Read the model definition and answer for the solid it produces. Units are mm, in the model's axes. Face numbers are marked on the shaded views. A direction names the side the tool comes from. Coordinates: 2 decimals unless noted, no trailing zeros. Write each loop counter-clockwise with the first axis right and the second up, starting at its lowest first coordinate (ties: lowest second). Pieces come first, ordered by that corner, then holes. Notation, with made-up numbers: M 64,13.5 L 100,13.5 A21 ccw 100,30.5 Z; hole C -32.75,51.25 d4. An arc over 180 degrees is marked long. Use a Markdown table: item, result. Add a question column.
from build123d import *

# Parameters (mm, degrees)
SKETCH4_R                               = 5
CUT_EXTRUDE1_DEPTH                      = 106.234262481
CBORE_FOR_M8_HEX_HEAD_BOLT1_D           = 8.4
CBORE_FOR_M8_HEX_HEAD_BOLT1_DEPTH       = 28.41
CBORE_FOR_M8_HEX_HEAD_BOLT1_CBORE_D     = 18.01
CBORE_FOR_M8_HEX_HEAD_BOLT1_CBORE_DEPTH = 5.68
CBORE_FOR_M8_HEX_HEAD_BOLT1_TIP         = 2.5236146
CHAMFER1_SIZE                           = 5
SKETCH8_R                               = 10
CUT_EXTRUDE2_DEPTH                      = 15
CIRPATTERN1_COUNT                       = 9


with BuildPart() as part:
    # Sketch2 → Revolve1 (revolve)
    with BuildSketch(Plane(origin=(0, 0, 0), x_dir=(1, 0, 0), z_dir=(0, 1, 0))):
        Polygon((49, 0), (71, 0), (71, 12), (51, 12), (51, 27), (31, 27), (31, 25), (31, 9), (28, 9), (25, -13.5), (27.5, -13.5), (27.5, -26.5), (27.5, -31.5), (47, -31.5), (47, -9.5), (47, -2), (47, 0), align=None)
    revolve(axis=Axis((0, 0, 21.110532956), (0, 0, -1)))

    # Sketch4 → Cut-Extrude1 (cut, through all)
    with BuildSketch(Plane.XY):
        with Locations((29, -50.229473419)):
            Circle(SKETCH4_R)
        with Locations((29, 50.22947342)):
            Circle(SKETCH4_R)
        with Locations((-58, 0)):
            Circle(SKETCH4_R)
    extrude(amount=-CUT_EXTRUDE1_DEPTH, mode=Mode.SUBTRACT)

    # CBORE for M8 Hex Head Bolt1
    with Locations(Plane.XY):
        with Locations((-10.071594305, 57.118849675), (-44.430577701, 37.281681362), (-44.430577701, -37.281681362), (-10.071594305, -57.118849675), (54.502172006, -19.837168313), (54.502172006, 19.837168313)):
            CounterBoreHole(CBORE_FOR_M8_HEX_HEAD_BOLT1_D / 2, CBORE_FOR_M8_HEX_HEAD_BOLT1_CBORE_D / 2, CBORE_FOR_M8_HEX_HEAD_BOLT1_CBORE_DEPTH, depth=CBORE_FOR_M8_HEX_HEAD_BOLT1_DEPTH)
            with Locations((0, 0, -(CBORE_FOR_M8_HEX_HEAD_BOLT1_DEPTH + CBORE_FOR_M8_HEX_HEAD_BOLT1_TIP / 2))):  # 118° drill point
                Cone(0, CBORE_FOR_M8_HEX_HEAD_BOLT1_D / 2, CBORE_FOR_M8_HEX_HEAD_BOLT1_TIP, mode=Mode.SUBTRACT)

    # Sketch7 → Cut-Revolve1 (revolve, cut)
    with BuildSketch(Plane(origin=(0, 0, 0), x_dir=(1, 0, 0), z_dir=(0, 1, 0)), mode=Mode.PRIVATE) as cut_revolve1_sk:
        Polygon((47, -9.5), (47, -7.5), (35, -7.5), (35, -8.5), (36, -8.5), (36, -31.5), (67.825, -31.5), (67.825, -9.5), align=None)
    revolve(cut_revolve1_sk.sketch.rotate(Axis((0, 0, 7.5), (0, 0, 1)), 180), axis=Axis((0, 0, 7.5), (0, 0, 1)), mode=Mode.SUBTRACT)

    # Chamfer1
    chamfer1_edges = [part.edges().sort_by_distance(p)[0] for p in [
        (36, 0, 31.5),
    ]]
    chamfer(chamfer1_edges, length=CHAMFER1_SIZE)

    # Sketch8 → Cut-Extrude2 (cut)
    with BuildSketch(Plane(origin=(0, 0, -27), x_dir=(-1, 0, 0), z_dir=(0, 0, -1))):
        with Locations((44.430577701, 37.281681362)):
            Circle(SKETCH8_R)
    cut_extrude2 = extrude(amount=-CUT_EXTRUDE2_DEPTH, mode=Mode.SUBTRACT)

    # CirPattern1: Cut-Extrude2 ×9 about axis, 3 skipped
    cirpattern1_axis = Axis((0, 0, -12), (0, 0, 1))
    add([cut_extrude2.rotate(cirpattern1_axis, i * 360 / CIRPATTERN1_COUNT) for i in range(1, CIRPATTERN1_COUNT) if i not in (1, 4, 7)], mode=Mode.SUBTRACT)


solid = part.part
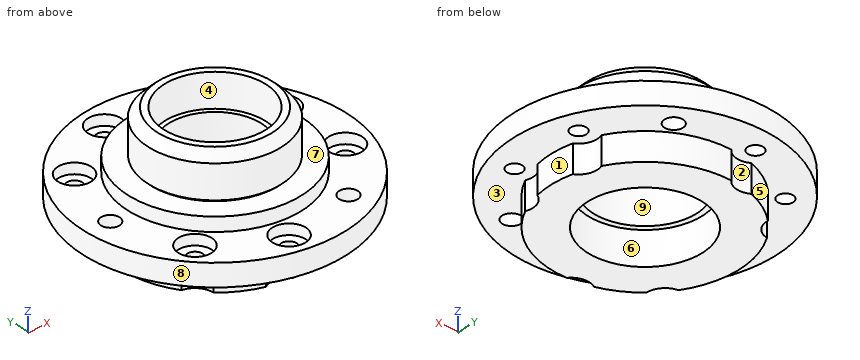
Item 1: Find section C-C on y = 0. Count the separate pieces of the cut face and the enclosed holes in it, then the cut area to 3 significant figures.
Item 2: Find section B-B on x = -58. Give the vertices of the cut face in (y, z).
Item 3: Each of these flat-tipped pins is pushed along its axis until it touches: pin 1 (11 mm diameter, centred on x = 54.5, y = 19.84, fed in from -Z); pin 2 (14.5 mm diameter, centred on x = 55.5, y = -17.5, fed in from +Z); pin 3 (9 mm diameter, centred on x = -9.5, y = -59, fed in from +Z). Where does it stop, or does it pass through?
Item 4: Determine the mould class of the marked faces 6, 7, 8 and 9 for opening direction X: pulls with the +X half, pulls with the -X half, needs draft (parallel to the pull), parting line crosses it, or undercut.
Item 5: For the marked faces 1, 2, 3, 4 and 5, determine the directions among +Z, -Z, +X, -X, +Y, -Y from which every point of the face is accessible in a straight line to the end or side of a thin tool.
Item 6: Find section A-A on z = -16. Give the vertices of the cut face in (x, y).
Item 7: Consider probe 1 along Y at (x, z) = (55.5, -6.5); probe 2 along Z at (x, y) = (27.5, -60); probe 3 along Z at (x, y) = (-35, -28). Determine where each line is inside the solid, lowest interval first.
Geometry says:
| question | item | result |
|---|---|---|
| 1 | separate pieces | 3 |
| 1 | enclosed holes | 0 |
| 1 | area | 2,220 mm2 |
| 2 | outline | M -40.95,-12 L -5,-12 L -5,0 L -40.95,0 Z; M 5,-12 L 40.95,-12 L 40.95,0 L 5,0 Z |
| 3 | pin 1 | stops at z = -12 |
| 3 | pin 2 | stops at z = 0 |
| 3 | pin 3 | stops at z = -5.68 |
| 4 | face 6 | undercut |
| 4 | face 7 | needs draft |
| 4 | face 8 | parting line crosses it |
| 4 | face 9 | undercut |
| 5 | face 1 | -Z, +X |
| 5 | face 2 | -Z, +Y |
| 5 | face 3 | -Z |
| 5 | face 4 | +Z |
| 5 | face 5 | -Z, -X, +Y |
| 6 | outline | M -43.03,-27.38 A10 cw -34.44,-37.62 A51 ccw -15.36,-48.63 A10 cw -2.2,-50.95 A51 ccw 45.23,-23.57 A10 cw 49.8,-11.01 A51 ccw 49.8,11.01 A10 cw 45.23,23.57 A51 ccw -2.2,50.95 A10 cw -15.36,48.63 A51 ccw -34.44,37.62 A10 cw -43.03,27.38 A51 ccw Z; hole C 0,0 d62 |
| 7 | probe 1 | y = -44.28 to -23.92, -15.76 to 15.76, 23.92 to 44.28 |
| 7 | probe 2 | z = -12 to 0 |
| 7 | probe 3 | z = -27 to 7.5 |
